Design review of the part shown in the three views and the two pictorial views. Dimensions are in mm from the part's minimum x, y and z. A direction names the side the tool comes from. Coordinates: 2 decimals unless noted, no trailing zeros. Loops run counter-clockwise (first coordinate to the right, second up) from the corner with the lowest first, then second, coordinate; pieces in that order, holes last. Notation, with made-up numbers: (-9, 60) -> (49, 60) arc R16 cw to (49, 66) -> close; hole circle Ø10 at (43.5, -28). An arc over 180 degrees is marked (long way). Answer in a Markdown table with one row per item.
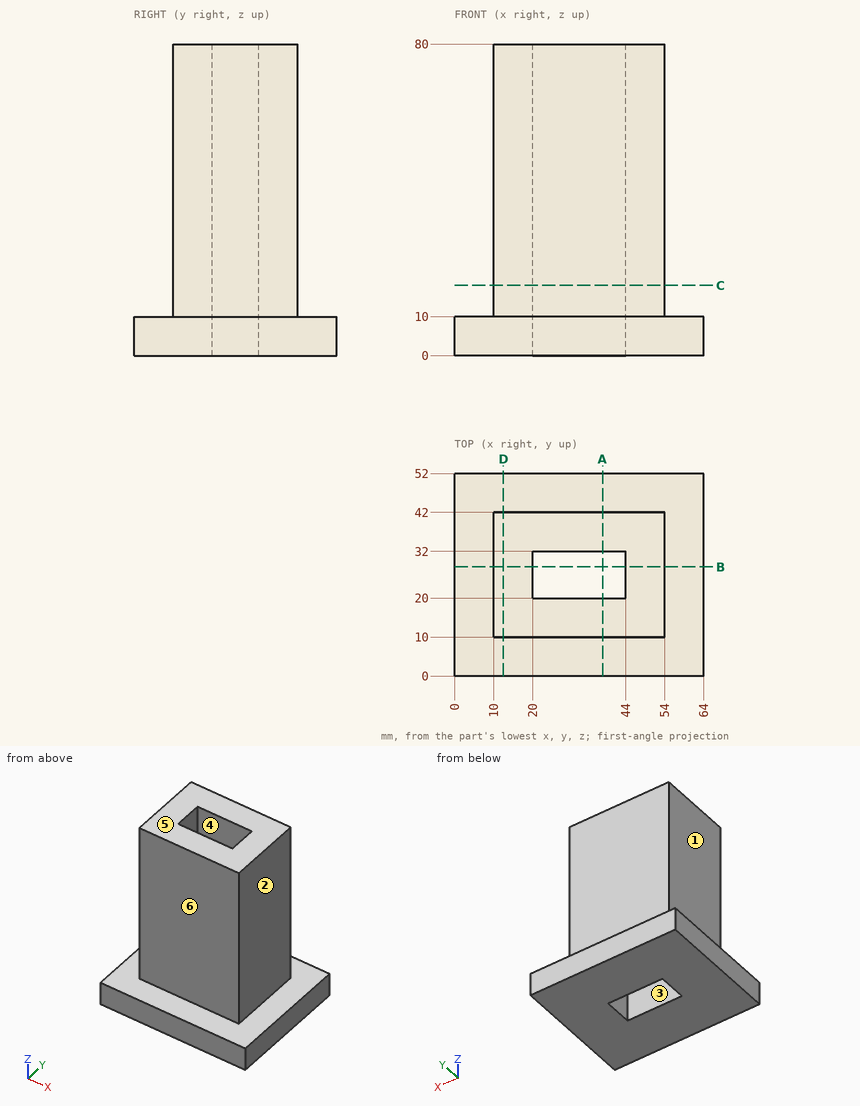
(1) For pin 1 (12 mm diameter, centred on y = 42.5, z = 69.5, fed in from +X); pin 2 (13 mm diameter, centred on x = 30, z = 28, fed in from -Y); pin 3 (6 mm diameter, centred on y = 24.5, z = 44, fed in from -X), all flat-tipped, find the tip position at first contact; note any pin that passes through.
Evaluation:
| item | result |
|---|---|
| pin 1 | stops at x = 54 |
| pin 2 | stops at y = 10 |
| pin 3 | stops at x = 10 |
(2) Draft analysis for pull direction Y (two halves, no side actions). For the marked faces 4, 5 and 6, state which applies: pulls with the +Y half, pulls with the -Y half, needs draft (parallel to the pull), parting line crosses it, or undercut.
Evaluation:
| item | result |
|---|---|
| face 4 | undercut |
| face 5 | needs draft |
| face 6 | pulls with the -Y half |
(3) Take a section at C-C on z = 18. Give the boundary of the cut face in (x, y), and give its area (3 significant figures).
Evaluation:
| item | result |
|---|---|
| outline | (10, 10) -> (54, 10) -> (54, 42) -> (10, 42) -> close; hole (20, 20) -> (44, 20) -> (44, 32) -> (20, 32) -> close |
| area | 1,120 mm² |
(4) Take a section at A-A on x = 38. Give the boundary of the cut face in (y, z), and give its area (3 significant figures).
Evaluation:
| item | result |
|---|---|
| outline | (0, 0) -> (20, 0) -> (20, 80) -> (10, 80) -> (10, 10) -> (0, 10) -> close; (32, 0) -> (52, 0) -> (52, 10) -> (42, 10) -> (42, 80) -> (32, 80) -> close |
| area | 1,800 mm² |
(5) Tool access review of the marked faces 1, 2 and 3: name each direction out of +Z, -Z, +X, -X, +Y, -Y from which nothing blocks a thin tool from reaching the whole face with its end or side.
Evaluation:
| item | result |
|---|---|
| face 1 | +Z, -X, +Y, -Y |
| face 2 | +Z, +X, +Y, -Y |
| face 3 | +Z, -Z |
(6) To check wall thickness, follow probe 1 along Y at (x, z) = (41, 44.5); probe 2 along X at (y, z) = (22, 40); probe 3 along Z at (x, y) = (57, 42). State the ranges of each line that lie inside material, in increasing order.
Evaluation:
| item | result |
|---|---|
| probe 1 | y = 10 to 20, 32 to 42 |
| probe 2 | x = 10 to 20, 44 to 54 |
| probe 3 | z = 0 to 10 |
(7) Take a section at B-B on y = 28. Give the boundary of the cut face in (x, z), and give its area (3 significant figures).
Evaluation:
| item | result |
|---|---|
| outline | (0, 0) -> (20, 0) -> (20, 80) -> (10, 80) -> (10, 10) -> (0, 10) -> close; (44, 0) -> (64, 0) -> (64, 10) -> (54, 10) -> (54, 80) -> (44, 80) -> close |
| area | 1,800 mm² |
(8) Take a section at D-D on x = 12.5. Give the boundary of the cut face in (y, z), and give its area (3 significant figures).
Evaluation:
| item | result |
|---|---|
| outline | (0, 0) -> (52, 0) -> (52, 10) -> (42, 10) -> (42, 80) -> (10, 80) -> (10, 10) -> (0, 10) -> close |
| area | 2,760 mm² |
